Can you work these out from the model? Positions are in its coordinate system, mm. A direction names the side the tool comes from. Coordinates: 2 decimals unless noted, no trailing zeros. Write each loop counter-clockwise with the first axis right and the second up, starting at its lowest first coordinate (ties: lowest second). Pieces come first, ordered by that corner, then holes. Notation, with made-up numbers: M 43.25,77.25 L 68.25,77.25 A27 ccw 68.25,110.25 Z; hole C 20.5,26.5 d10. An arc over 180 degrees is marked long. Use one line per item in the form item = value. Start each with the question number.
```python
from build123d import *

# Parameters (mm, degrees)
SKETCH1_R           = 14
BOSS_EXTRUDE1_DEPTH = 19
SKETCH2_R           = 4.5
BOSS_EXTRUDE2_DEPTH = 1.5
SKETCH3_R           = 2.5
BOSS_EXTRUDE3_DEPTH = 2.5
SKETCH4_R           = 2.5
BOSS_EXTRUDE4_DEPTH = 6
CHAMFER1_SIZE       = 0.25
BOSS_EXTRUDE5_START = -0.5
SKETCH6_R           = 1.05
BOSS_EXTRUDE5_DEPTH = 0.5
CUT_EXTRUDE1_DEPTH  = 6
SKETCH8_W           = 14.6
SKETCH8_H           = 17
BOSS_EXTRUDE6_DEPTH = 2
SKETCH9_R           = 0.7
BOSS_EXTRUDE7_DEPTH = 9


with BuildPart() as part:
    # Sketch1 → Boss-Extrude1 (new body)
    with BuildSketch(Plane(origin=(0, 0, 0), x_dir=(1, 0, 0), z_dir=(0, 1, 0))):
        with Locations(Location((0, 0, 0), (0, 0, 270))):
            Circle(SKETCH1_R)
    extrude(amount=BOSS_EXTRUDE1_DEPTH)

    # Sketch2 → Boss-Extrude2 (add)
    with BuildSketch(Plane(origin=(0, 19, 0), x_dir=(1, 0, 0), z_dir=(0, 1, 0))):
        with Locations(Location((0, 8, 0), (0, 0, 270))):
            Circle(SKETCH2_R)
    extrude(amount=BOSS_EXTRUDE2_DEPTH)

    # Sketch3 → Boss-Extrude3 (add)
    with BuildSketch(Plane(origin=(0, 20.5, 0), x_dir=(1, 0, 0), z_dir=(0, 1, 0))):
        with Locations(Location((0, 8, 0), (0, 0, 270))):
            Circle(SKETCH3_R)
    extrude(amount=BOSS_EXTRUDE3_DEPTH)

    # Sketch4 → Boss-Extrude4 (add)
    with BuildSketch(Plane(origin=(0, 23, 0), x_dir=(1, 0, 0), z_dir=(0, 1, 0))):
        with Locations(Location((0, 8, 0), (0, 0, 270))):
            Circle(SKETCH4_R)
    extrude(amount=BOSS_EXTRUDE4_DEPTH)

    # Chamfer1
    chamfer1_edges = [part.edges().sort_by_distance(p)[0] for p in [
        (0, 29, -10.5),
    ]]
    chamfer(chamfer1_edges, length=CHAMFER1_SIZE)

    # Sketch6 → Boss-Extrude5 (add)
    # profile 1 of 2: a face of its own
    with BuildSketch(Plane(origin=(0, 19, 0), x_dir=(1, 0, 0), z_dir=(0, 1, 0)).offset(BOSS_EXTRUDE5_START)):
        with BuildLine():
            Line((-13.555441712, 3.5), (-17.5, 3.5))
            ThreePointArc((-17.5, 3.5), (-21, 0), (-17.5, -3.5))
            Line((-17.5, -3.5), (-13.555441712, -3.5))
            ThreePointArc((-13.555441712, -3.5), (-14, 0), (-13.555441712, 3.5))
        make_face()
        with Locations(Location((-17.5, 0, 0), (0, 0, 270))):
            Circle(SKETCH6_R, mode=Mode.SUBTRACT)
    # profile 2 of 2: a face of its own
    with BuildSketch(Plane(origin=(0, 19, 0), x_dir=(1, 0, 0), z_dir=(0, 1, 0)).offset(BOSS_EXTRUDE5_START)):
        with BuildLine():
            Line((17.5, 3.5), (13.555441712, 3.5))
            ThreePointArc((13.555441712, 3.5), (13.888415748, 1.764060095), (14, 0))
            ThreePointArc((14, 0), (13.888415748, -1.764060095), (13.555441712, -3.5))
            Line((13.555441712, -3.5), (17.5, -3.5))
            ThreePointArc((17.5, -3.5), (21, 0), (17.5, 3.5))
        make_face()
        with BuildLine():
            ThreePointArc((16.45, 0), (17.5, 1.05), (18.55, 0))
            ThreePointArc((18.55, 0), (17.5, -1.05), (16.45, 0))
        make_face(mode=Mode.SUBTRACT)
    extrude(amount=BOSS_EXTRUDE5_DEPTH)

    # Sketch7 → Cut-Extrude1 (cut)
    with BuildSketch(Plane(origin=(0, 29, 0), x_dir=(1, 0, 0), z_dir=(0, 1, 0))):
        Polygon((0, 9.5), (-3.852733209, 9.5), (-3.852733209, 12.808282557), (3.692444336, 12.808282557), (3.692444336, 9.5), align=None)
        Polygon((3.692444336, 6.5), (0, 6.5), (-3.852733209, 6.5), (-3.852733209, 3.191717443), (3.692444336, 3.191717443), align=None)
    extrude(amount=-CUT_EXTRUDE1_DEPTH, mode=Mode.SUBTRACT)

    # Sketch8 → Boss-Extrude6 (add)
    with BuildSketch(Plane(origin=(0, 19, 0), x_dir=(1, 0, 0), z_dir=(0, 1, 0))):
        with Locations((0, -8.5)):
            Rectangle(SKETCH8_W, SKETCH8_H)
    extrude(amount=-BOSS_EXTRUDE6_DEPTH)

    # Sketch9 → Boss-Extrude7 (add)
    with BuildSketch(Plane.XY.offset(17)):
        with Locations((-1.645828478, 18)):
            Circle(SKETCH9_R)
        with Locations((1.645828478, 18)):
            Circle(SKETCH9_R)
        with Locations((5.295828478, 18)):
            Circle(SKETCH9_R)
        with Locations((-5.295828478, 18)):
            Circle(SKETCH9_R)
    extrude(amount=BOSS_EXTRUDE7_DEPTH)


solid = part.part
```
1) Suppose I cut it at A-A on z = 0. Please give me the cut outline in (x, y), and give its area (3 significant figures).
2) Please list where these lines run through material, in increasing order: line 1 (Z direction, x = 17.5, y = 18.8); line 2 (Z direction, x = 2, y = 26.5); line 3 (Y direction, x = 9, z = -7.5).
3) Suppose I cut it at D-D on x = -10.5. Please give me the cut outline in (y, z), and give its area (3 significant figures).
4) Will these pins go through, and if not, where does the flat tip stop? pin 1 Ø5 at (y, z) = (4, -9) entering from -X; pin 2 Ø12 at (y, z) = (15.5, 15) entering from +X; pin 3 Ø2.5 at (x, z) = (17.5, 0) entering from -Y; pin 4 Ø1.7 at (x, z) = (-17.5, 0) entering from +Y.
5) Suppose I cut it at B-B on z = 21. Please give me the cut outline in (x, y), and give its area (3 significant figures).
6) Suppose I cut it at C-C on y = 23.75. Please give me the cut outline in (x, z).
7) Which directions (+Z, -Z, +X, -X, +Y, -Y) give clear straight access to the entire face, cutting with the end or side of a thin tool? Please do faces 1 (the face through (-2, 20.5, -6)), 2 (the face through (0, 26, -6.5)), 3 (the face through (0, 23, -10)), 4 (the face through (-5.387, 18.694, 21.437)).
8) If we mould it in two halves opening along X, with no side actions, what happens to faces 5 (the face through (-1.737, 18.694, 21.437)), 6 (the face through (16.45, 18.75, 0.05)), 7 (the face through (2, 18, 26)), 8 (the face through (7.3, 18, 15))? For each: +X half, -X half, draft (parallel to the pull), parting line (faces both ways), or undercut.
Computed values:
q1.outline = M -21,18.5 L -18.55,18.5 L -18.55,19 L -21,19 Z; M -16.45,18.5 L -14,18.5 L -14,0 L 14,0 L 14,18.5 L 16.45,18.5 L 16.45,19 L -16.45,19 Z; M 18.55,18.5 L 21,18.5 L 21,19 L 18.55,19 Z
q1.area = 537 mm²
q2.line_1 = -3.5 to -1.05, 1.05 to 3.5
q2.line_2 = -9.5 to -6.5
q2.line_3 = 0 to 19
q3.outline = M 0,-9.26 L 19,-9.26 L 19,9.26 L 0,9.26 Z
q3.area = 352 mm²
q4.pin_1 = -12.4
q4.pin_2 = 10.72
q4.pin_3 = 18.5
q4.pin_4 = through
q5.outline = C -5.3,18 d1.4; C -1.65,18 d1.4; C 1.65,18 d1.4; C 5.3,18 d1.4
q5.area = 6.16 mm²
q6.outline = M -2,-9.5 L 2,-9.5 A2.5 ccw 2,-6.5 L -2,-6.5 A2.5 ccw Z
q7.face_1 = +Y
q7.face_2 = +Z, +X, -X, +Y
q7.face_3 = -Z, +X, -X, +Y
q7.face_4 = +Z
q8.face_5 = undercut
q8.face_6 = undercut
q8.face_7 = draft
q8.face_8 = +X half
